Source: three-view drawing plus pictorial views. Frame: mm from the lowest corner of the part. Round coordinates to 2 decimals unless told otherwise and drop trailing zeros. Loops run counter-clockwise (first coordinate to the right, second up) from the corner with the lowest first, then second, coordinate; pieces in that order, holes last. Notation, with made-up numbers: (-29.5, 27.25) -> (29.5, 27.25) arc R21 cw to (29.5, 48.25) -> close; hole circle Ø5 at (75, 7.25). An arc over 180 degrees is marked (long way). Answer in a Markdown table with one row per item.
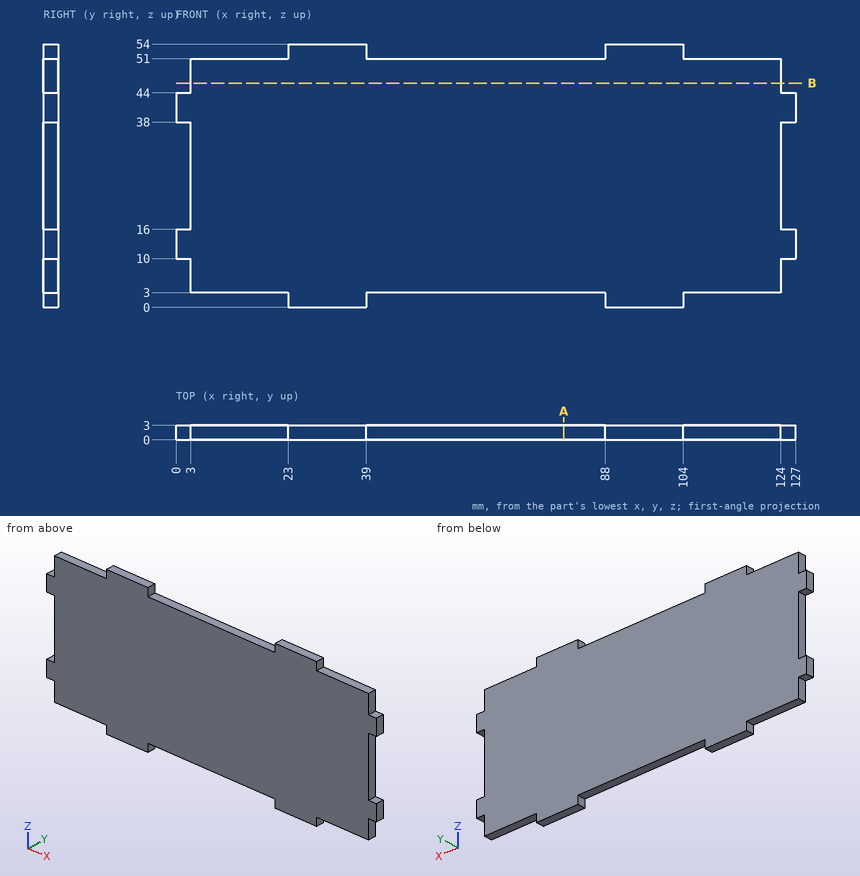
Item 1: Line query: probe 1 along X at (y, z) = (0.65, 47.5); probe 2 along Z at (x, y) = (72.5, 0.9); probe 3 along X at (y, z) = (1.25, 51.5). Output: solid intervals per line, ascending. Write a range as [from, to].
Answer:
| item | result |
|---|---|
| probe 1 | x = [3, 124] |
| probe 2 | z = [3, 51] |
| probe 3 | x = [23, 39], [88, 104] |
Item 2: Cut plane B-B (z = 46). Output: boundary loops of the cut face in (x, y).
Answer:
| item | result |
|---|---|
| outline | (3, 0) -> (124, 0) -> (124, 3) -> (3, 3) -> close |
Item 3: Pin query (flat end, axial travel): pin 1 Ø1.5 at (x, y) = (1.5, 1.5) entering from -Z; pin 2 Ø1 at (x, z) = (109.5, 13) entering from -Y; pin 3 Ø1.5 at (y, z) = (1, 1) entering from -X; pin 4 Ø0.9 at (y, z) = (1, 5) entering from +X. Return the tip coordinate at first contact, or that it passes through.
Answer:
| item | result |
|---|---|
| pin 1 | stops at z = 10 |
| pin 2 | stops at y = 0 |
| pin 3 | stops at x = 23 |
| pin 4 | stops at x = 124 |
Item 4: Cut plane A-A (x = 79.5). Output: boundary loops of the cut face in (y, z).
Answer:
| item | result |
|---|---|
| outline | (0, 3) -> (3, 3) -> (3, 51) -> (0, 51) -> close |
